Can you work these out from the model? Positions are in its coordinate system, mm. Give positions to 0.01 mm unless a question says otherwise; leave off trailing zeros. Loops run counter-clockwise (first coordinate to the right, second up) from the corner with the lowest first, then second, coordinate; pieces in that order, holes last. Notation, with made-up numbers: (87.25, 82.5) -> (130.25, 82.5) arc R28 cw to (130.25, 107.5) -> close; hole circle Ø10 at (5.25, -35). An arc over 180 degrees is marked (long way). Return JSON: item names as keys, results as strings. Group by question number.
Q1. Suppose I cut it at D-D, the plane z = 4.2. Count the separate pieces of the cut face and the enclosed holes in it, and give its area (3 significant figures).
Q2. Suppose I cut it at A-A, the plane x = 0. Please give me the cut outline in (y, z).
Q3. Suppose I cut it at C-C, the plane x = -35.5. Please give me the cut outline in (y, z), and give its area (3 significant figures).
Q4. Will these pins go through, and if not, where does the flat tip stop? pin 1 (1.5 mm diameter, centred on x = -5, z = 2.5, fed in from +Y); pin 2 (8 mm diameter, centred on x = -0.5, y = -49, fed in from -Z); pin 3 (3 mm diameter, centred on y = -8.5, z = 4, fed in from -X); pin 4 (10 mm diameter, centred on x = 29.5, y = 14.5, fed in from -Z).
Q5. I need wall thicknesses on line 1 along Y through (x, z) = (0, 2.05); line 2 along X through (y, z) = (37, 2.1); line 3 along Y through (x, z) = (-13, 2.25). Which ranges of each line are inside material? Lowest first, please. Write a range as [from, to].
Q6. Suppose I cut it at B-B, the plane y = 20. Please give me the cut outline in (x, z), and give its area (3 significant figures).
Solid Edge part; units mm, degrees
sketch "Sketch1" plane through (0, 0, 0) normal (0, 0, 1) x (1, 0, 0)
  circle A0 centre (0, 0) radius 62.5
extrude "Protrusion1" add sketch "Sketch1" along normal blind 5
sketch "Sketch2" plane through (0, 0, 5) normal (0, 0, 1) x (1, 0, 0)
  circle A0 centre (15, -42.5) radius 1.95
  circle A1 centre (-15, -42.5) radius 1.95
  circle A2 centre (-15, 42.5) radius 1.95
  circle A3 centre (15, 42.5) radius 1.95
extrude "Cutout1" cut sketch "Sketch2" against normal through all
sketch "Sketch3" plane through (0, 0, 5) normal (0, 0, 1) x (1, 0, 0)
  line L0 (-15, -35) -> (-25, -43.3013)
  arc A0 (-25, -43.3013) -> (-25, 43.3013) centre (0, 0) cw
  line L1 (-25, 43.3013) -> (-15, 35)
  line L2 (-15, 35) -> (15, 35)
  line L3 (25, 43.3013) -> (15, 35)
  line L4 (15, -35) -> (25, -43.3013)
  line L5 (15, -35) -> (-15, -35)
  arc A1 (25, 43.3013) -> (25, -43.3013) centre (0, 0) cw
extrude "Cutout2" cut sketch "Sketch3" against normal through all
fillet "Round_1" radius 5 8 edges at (-15, 35, 2.5) (15, 35, 2.5) (25, 43.3013, 2.5) (25, -43.3013, 2.5) (15, -35, 2.5) (-15, -35, 2.5) (-25, -43.3013, 2.5) (-25, 43.3013, 2.5)
sketch "Sketch4" plane through (0, 0, 5) normal (0, 0, 1) x (1, 0, 0)
  circle A0 centre (-39.7748, 39.7748) radius 1
  circle A1 centre (39.7748, 39.7748) radius 1
  circle A2 centre (39.7748, -39.7748) radius 1
  circle A3 centre (-39.7748, -39.7748) radius 1
extrude "Cutout3" cut sketch "Sketch4" against normal through all
sketch "Sketch5" plane through (0, 0, 5) normal (0, 0, 1) x (1, 0, 0)
  line L0 (-20, -5) -> (-56.0273, -5)
  line L1 (-56.0273, -5) -> (-56.0273, 5)
  line L2 (-56.0273, 5) -> (-20, 5)
  line L3 (-20, 5) -> (-20, 15)
  line L4 (-20, 15) -> (20, 15)
  line L5 (20, 15) -> (20, 5)
  line L6 (20, 5) -> (56.0273, 5)
  line L7 (56.0273, 5) -> (56.0273, -5)
  line L8 (56.0273, -5) -> (20, -5)
  line L9 (20, -5) -> (20, -15)
  line L10 (20, -15) -> (-20, -15)
  line L11 (-20, -15) -> (-20, -5)
extrude "Protrusion2" add sketch "Sketch5" against normal up to vertex (5 mm away)
fillet "Round_4" radius 10 4 edges at (-20, -15, 2.5) (20, -15, 2.5) (20, 15, 2.5) (-20, 15, 2.5)
fillet "Round_4" radius 2 4 edges at (-49.7494, -5, 2.5) (-49.7494, 5, 2.5) (49.7494, -5, 2.5) (49.7494, 5, 2.5)
sketch "Sketch6" plane through (0, 0, 5) normal (0, 0, 1) x (1, 0, 0)
  circle A0 centre (-8.5, 0) radius 6
  circle A1 centre (8.5, 0) radius 6
extrude "Cutout4" cut sketch "Sketch6" against normal through all
fillet "Round_5" radius 10 4 edges at (20, -5, 2.5) (20, 5, 2.5) (-20, 5, 2.5) (-20, -5, 2.5)
Ans:
{
 "1": {"separate pieces": "1", "enclosed holes": "12", "area": "7,010 mm^2"},
 "2": {"outline": "(-62.5, 0) -> (-35, 0) -> (-35, 5) -> (-62.5, 5) -> close; (-15, 0) -> (15, 0) -> (15, 5) -> (-15, 5) -> close; (35, 0) -> (62.5, 0) -> (62.5, 5) -> (35, 5) -> close"},
 "3": {"outline": "(-51.44, 0) -> (-35.21, 0) -> (-35.21, 5) -> (-51.44, 5) -> close; (-5, 0) -> (5, 0) -> (5, 5) -> (-5, 5) -> close; (35.21, 0) -> (51.44, 0) -> (51.44, 5) -> (35.21, 5) -> close", "area": "212 mm^2"},
 "4": {"pin 1": "stops at y = 62.36", "pin 2": "stops at z = 0", "pin 3": "stops at x = -62.11", "pin 4": "passes through"},
 "5": {"line 1": "y = [-62.5, -35], [-15, 15], [35, 62.5]", "line 2": "x = [-50.37, -33.63], [-17.41, 17.41], [33.63, 50.37]", "line 3": "y = [-61.13, -35], [-14.54, -3.97], [3.97, 14.54], [35, 61.13]"},
 "6": {"outline": "(-59.21, 0) -> (-45.83, 0) -> (-45.83, 5) -> (-59.21, 5) -> close; (45.83, 0) -> (59.21, 0) -> (59.21, 5) -> (45.83, 5) -> close", "area": "134 mm^2"}
}
